Could you check a few things on this drawing? It's one solid part, dimensions in mm from its lowest x, y, z. A direction names the side the tool comes from. Coordinates: 2 decimals unless noted, no trailing zeros. Write each loop counter-clockwise with the first axis right and the second up, starting at its lowest first coordinate (ties: lowest second). Pieces come first, ordered by that corner, then holes. Notation, with made-up numbers: (-36, 31.25) - (-23, 31.25) arc R20 ccw to (-23, 62.25) - close; hole circle Ø1 at (-23, 3.5). An arc over 180 degrees is marked (long way). Use one line per item in the form item = value. Start each with the question number.
(1) Thinking about a two-plate mould opening in X: for the marked faces 1, 2 and 3, which applies, pulls with the +X half, pulls with the -X half, needs draft (parallel to the pull), parting line crosses it, or undercut?
(2) If we section it at A-A on y = 3.9: Please give me the cut outline in (x, z).
(3) For pin 1 Ø2 at (x, y) = (12.5, 4.5) entering from +Z; pin 2 Ø2 at (x, y) = (3, 4.25) entering from +Z; pin 3 Ø1 at (x, z) = (9, 0.5) entering from -Y; pin 4 Ø0.8 at (y, z) = (5.5, 0.5) entering from -X (3 decimals), each with a flat end and sliding along its axis, tell me the tip position at first contact or that it passes through.
(4) On a 3-axis mill with a long thin cutter (end or side, diameter ignored), from which of +Z, -Z, +X, -X, +Y, -Y can I reach the whole of each face in a straight line? I mean the marked faces 4 and 5. Say none if no direction works.
(5) If we section it at D-D on x = 11.75: Please give me the cut outline in (y, z).
(6) If we section it at B-B on y = 1.35: Please give me the cut outline in (x, z).
(7) If I drill on probe 1 along X at (y, z) = (4.25, 1.15); probe 2 along X at (y, z) = (5.65, 0.7); probe 3 along X at (y, z) = (1.1, 0.7), over which ranges is the centre line in solid material (lowest first)? Write a range as from..to.
(8) If we section it at C-C on z = 1.35: Please give me the cut outline in (x, y).
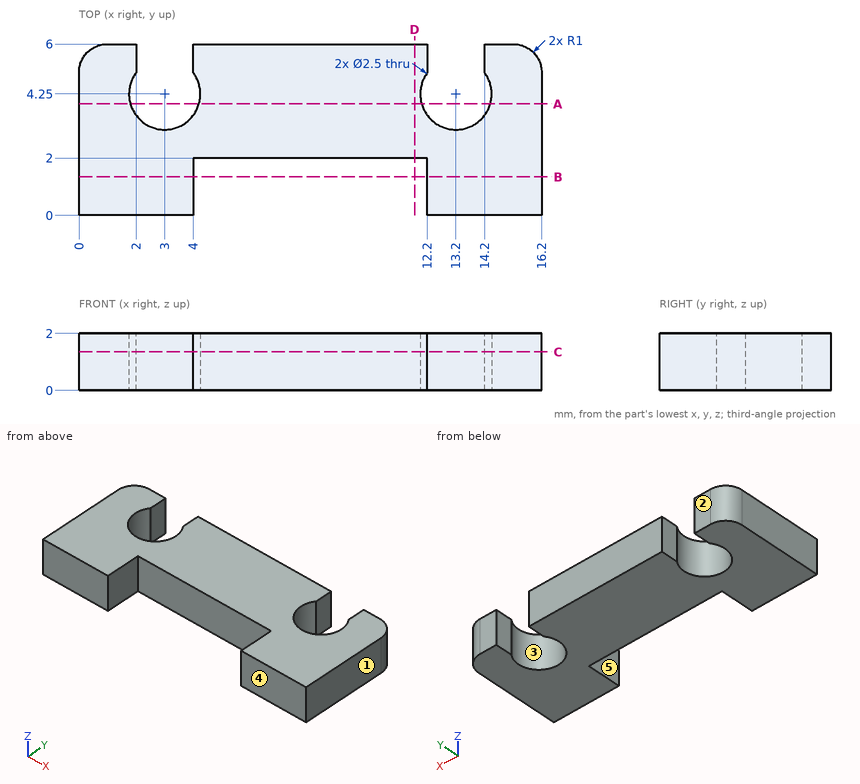
Reported:
q1.face_1 = pulls with the +X half
q1.face_2 = needs draft
q1.face_3 = undercut
q2.outline = (0, 0) - (1.8, 0) - (1.8, 2) - (0, 2) - close; (4.2, 0) - (12, 0) - (12, 2) - (4.2, 2) - close; (14.4, 0) - (16.2, 0) - (16.2, 2) - (14.4, 2) - close
q3.pin_1 = 2
q3.pin_2 = through
q3.pin_3 = 2
q3.pin_4 = 0.005
q4.face_4 = +Z, -Z, +X, -X, -Y
q4.face_5 = +Z, -Z, -Y
q5.outline = (2, 0) - (6, 0) - (6, 2) - (2, 2) - close
q6.outline = (0, 0) - (4, 0) - (4, 2) - (0, 2) - close; (12.2, 0) - (16.2, 0) - (16.2, 2) - (12.2, 2) - close
q7.probe_1 = 0..1.75, 4.25..11.95, 14.45..16.2
q7.probe_2 = 0.24..2, 4..12.2, 14.2..15.96
q7.probe_3 = 0..4, 12.2..16.2
q8.outline = (0, 0) - (4, 0) - (4, 2) - (12.2, 2) - (12.2, 0) - (16.2, 0) - (16.2, 5) arc R1 ccw to (15.2, 6) - (14.2, 6) - (14.2, 5) arc R1.25 cw (long way) to (12.2, 5) - (12.2, 6) - (4, 6) - (4, 5) arc R1.25 cw (long way) to (2, 5) - (2, 6) - (1, 6) arc R1 ccw to (0, 5) - close
